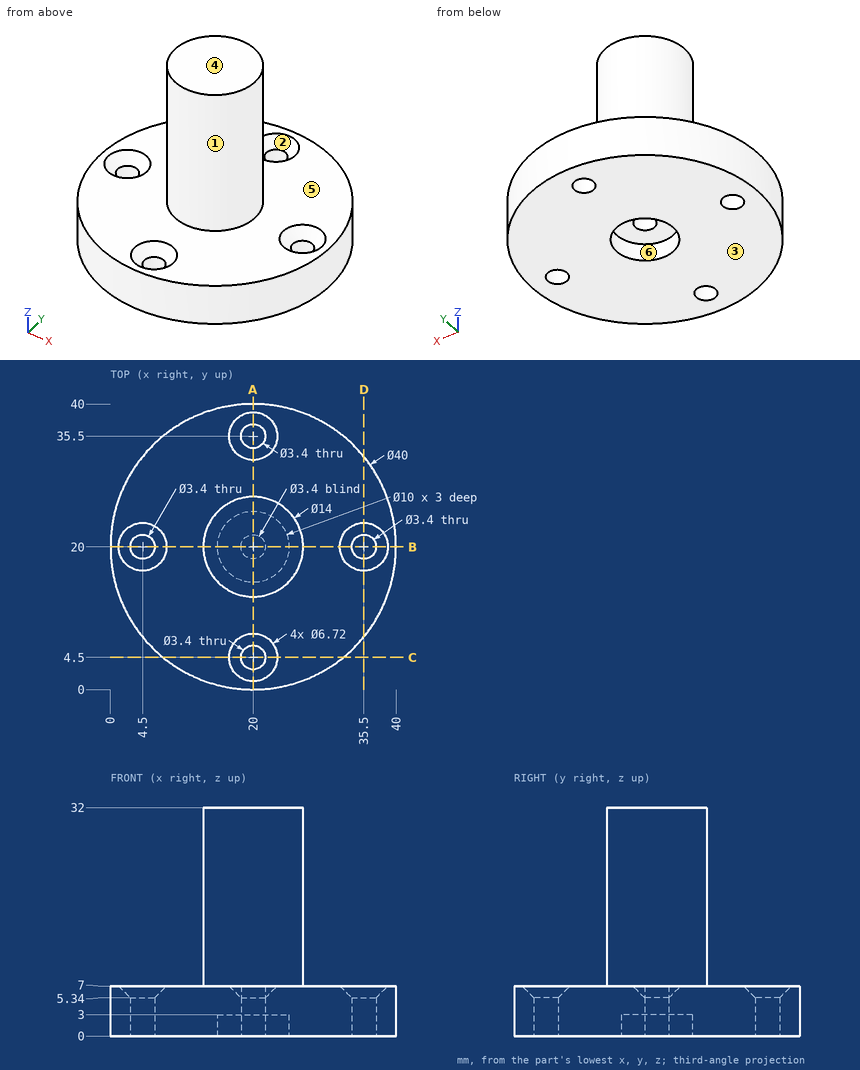
Can you work these out from the drawing? Everything is in mm from the part's minimum corner. A direction names the side the tool comes from. Give positions to 0.01 mm unless a question says otherwise; leave off trailing zeros. Loops run counter-clockwise (first coordinate to the right, second up) from the corner with the lowest first, then second, coordinate; pieces in that order, holes last. Notation, with made-up numbers: (-22, 52.25) - (33, 52.25) arc R29 ccw to (33, 83.25) - close; hole circle Ø3 at (-40, 18.5). An arc over 180 degrees is marked (long way). Use one line per item in the form item = value.
1. I want a section at A-A (x = 20). Please give me the cut outline in (y, z).
Response values:
outline = (0, 0) - (2.8, 0) - (2.8, 5.34) - (1.14, 7) - (0, 7) - close; (6.2, 0) - (15, 0) - (15, 3) - (18.3, 3) - (18.3, 7) - (21.7, 7) - (21.7, 3) - (25, 3) - (25, 0) - (33.8, 0) - (33.8, 5.34) - (32.14, 7) - (27, 7) - (27, 32) - (13, 32) - (13, 7) - (7.86, 7) - (6.2, 5.34) - close; (37.2, 0) - (40, 0) - (40, 7) - (38.86, 7) - (37.2, 5.34) - close
2. I want a section at C-C (y = 4.5). Please give me the cut outline in (x, z).
Response values:
outline = (7.36, 0) - (18.3, 0) - (18.3, 5.34) - (16.64, 7) - (7.36, 7) - close; (21.7, 0) - (32.64, 0) - (32.64, 7) - (23.36, 7) - (21.7, 5.34) - close
3. Thinking about a two-plate mould opening in X: for the marked faces 1, 2 and 3, which applies, released by +X, released by -X, zero draft, split by the parting line, or undercut?
Response values:
face_1 = split by the parting line
face_2 = undercut
face_3 = zero draft
4. I'm going to push flat-ended pins straight in: pin 1 Ø1 at (x, z) = (17.5, 15.5) entering from -Y; pin 2 Ø8 at (y, z) = (14.5, 15.5) entering from +X; pin 3 Ø5 at (x, y) = (33.5, 8) entering from +Z. Where does each tip first touch, or does it pass through?
Response values:
pin_1 = 13.29
pin_2 = 26.84
pin_3 = 7
5. On a 3-axis mill with a long thin cutter (end or side, diameter ignored), from which of +Z, -Z, +X, -X, +Y, -Y can I reach the whole of each face in a straight line? I mean the marked faces 4, 5 and 6. Say none if no direction works.
Response values:
face_4 = +Z, +X, -X, +Y, -Y
face_5 = +Z
face_6 = -Z
6. I need wall thicknesses on probe 1 along Y at (x, z) = (20, 3.5); probe 2 along Y at (x, z) = (20, 1); probe 3 along Y at (x, z) = (4, 3). Which ranges of each line are inside material? Lowest first, please.
Response values:
probe_1 = 0 to 2.8, 6.2 to 18.3, 21.7 to 33.8, 37.2 to 40
probe_2 = 0 to 2.8, 6.2 to 15, 25 to 33.8, 37.2 to 40
probe_3 = 8 to 18.38, 21.62 to 32
